Read the model definition and answer for the solid it produces. Units are mm, in the model's axes. Coordinates: 2 decimals unless noted, no trailing zeros. Loops run counter-clockwise (first coordinate to the right, second up) from the corner with the lowest first, then second, coordinate; pieces in that order, holes last.
Autodesk Inventor part; units mm, degrees
ref_plane "YZ Plane" through (0, 0, 0) normal (1, 0, 0) x (0, 1, 0)
ref_plane "XZ Plane" through (0, 0, 0) normal (0, 1, 0) x (-1, 0, 0)
ref_plane "XY Plane" through (0, 0, 0) normal (0, 0, 1) x (1, 0, 0)
sketch "Sketch1" plane through (0, 0, 0) normal (1, 0, 0) x (0, 1, 0)
  line L0 (0, 0) -> (360, 0)
  line L1 (360, 0) -> (360, -360)
  line L2 (360, -360) -> (0, -360)
  line L3 (0, -360) -> (0, -310)
  line L4 (0, -50) -> (310, -50)
  line L5 (310, -50) -> (310, -310)
  line L6 (310, -310) -> (0, -310)
  line L7 (0, -310) -> (0, -50)
  line L8 (0, -50) -> (0, 0)
  line L9 (0, -310) -> (0, -50)
  dimension "d4" = 360
  dimension "d5" = 360
  dimension "d6" = 310
  dimension "d7" = 260
extrude "Extrusion1" add sketch "Sketch1" along normal blind 3 contours L0 L1 L2 L3 L6 L5 L4 L8
hole "Hole1" at (3, 348, -12) direction (-1, 0, 0) diameter 4 end through all
hole "Hole2" at (3, 348, -348) direction (-1, 0, 0) diameter 4 end through all
hole "Hole3" at (3, 12, -348) direction (-1, 0, 0) diameter 4 end through all
hole "Hole4" at (3, 12, -12) direction (-1, 0, 0) diameter 4 end through all
properties part number "FrameCentre" material "Dibond Yellow"
Q1. A flat-ended cylindrical pin translates along its axis: pin 1 Ø0.9 at (x, z) = (2, -164) entering from -Y. Find the tip coordinate at first contact, or state that the pin passes through.
Findings below:
pin 1: stops at y = 310
Q2. A cutting plane is placed at C-C (z = -172.5). Give the vertices of the cut face in (x, y), then the cut area to 3 significant figures.
Findings below:
outline: (0, 310) - (3, 310) - (3, 360) - (0, 360) - close
area: 150 mm2
Q3. Straight lines are drawn through the part: probe 1 along Y at (x, z) = (1.15, -12); probe 2 along Z at (x, y) = (1.2, 239); probe 3 along Z at (x, y) = (1.15, 12). For each, find the intervals that lie inside material, in ascending order.
Findings below:
probe 1: y = 0 to 10, 14 to 346, 350 to 360
probe 2: z = -360 to -310, -50 to 0
probe 3: z = -360 to -350, -346 to -310, -50 to -14, -10 to 0
Q4. A cutting plane is placed at B-B (y = 163). Give the vertices of the cut face in (x, z), then the cut area to 3 significant figures.
Findings below:
outline: (0, -360) - (3, -360) - (3, -310) - (0, -310) - close; (0, -50) - (3, -50) - (3, 0) - (0, 0) - close
area: 300 mm2
Q5. A cutting plane is placed at A-A (x = 0.6). Give the vertices of the cut face in (y, z), then the cut area to 3 significant figures.
Findings below:
outline: (0, -360) - (360, -360) - (360, 0) - (0, 0) - (0, -50) - (310, -50) - (310, -310) - (0, -310) - close; hole circle Ø4 at (12, -348); hole circle Ø4 at (12, -12); hole circle Ø4 at (348, -348); hole circle Ø4 at (348, -12)
area: 48,900 mm2
